The listing builds one solid part. Answer for the finished solid, in the listing's coordinates (mm). A direction names the side the tool comes from. Round coordinates to 2 decimals unless told otherwise and drop trailing zeros. Write each loop counter-clockwise with the first axis right and the second up, starting at its lowest first coordinate (ties: lowest second). Pieces come first, ordered by that corner, then holes. Notation, with made-up numbers: (56.25, 51) - (71.25, 51) arc R24 ccw to (71.25, 85) - close; hole circle Ø10 at (31, 24). An arc over 180 degrees is marked (long way). Answer in a Markdown table with one row per item.
from build123d import *

# Parameters (mm, degrees)
BOSS_EXTRUDE1_DEPTH                          = 75
SKETCH2_R                                    = 1.3
CUT_EXTRUDE1_DEPTH                           = 34
CBORE_FOR_M3_HEX_SOCKET_HEAD_CAP_SCR_2_COUNT = 2
CBORE_FOR_M3_HEX_SOCKET_HEAD_CAP_SCR_2_PITCH = 60
CBORE_FOR_M3_HEX_SOCKET_HEAD_CAP_SCR_3_COUNT = 2
CBORE_FOR_M3_HEX_SOCKET_HEAD_CAP_SCR_3_PITCH = 57.567351858
CBORE_FOR_M3_HEX_SOCKET_HEAD_CAP_SCR_4_COUNT = 2
CBORE_FOR_M3_HEX_SOCKET_HEAD_CAP_SCR_4_PITCH = 17.720045147
FILLET2_R                                    = 12.5
BOSS_EXTRUDE2_START                          = 10
BOSS_EXTRUDE2_DEPTH                          = 10
CHAMFER3_SIZE                                = 0.5
BOSS_EXTRUDE3_START                          = 1.5
BOSS_EXTRUDE3_DEPTH                          = 1.5


with BuildPart() as part:
    # Sketch1 → Boss-Extrude1 (new body)
    with BuildSketch(Plane.XY):
        Polygon((0, 0), (60, 0), (60, 8.5), (30, 8.5), (0, 8.5), align=None)
    extrude(amount=BOSS_EXTRUDE1_DEPTH)

    # Sketch2 → Cut-Extrude1 (cut)
    with BuildSketch(Plane(origin=(0, 8.5, 0), x_dir=(1, 0, 0), z_dir=(0, 1, 0))):
        with Locations(Location((45, -64.5, 0), (0, 0, 180))):
            Circle(SKETCH2_R)
        with Locations(Location((45, -10.5, 0), (0, 0, 180))):
            Circle(SKETCH2_R)
    extrude(amount=-CUT_EXTRUDE1_DEPTH, mode=Mode.SUBTRACT)

    # Sketch4 → CBORE for M3 Hex Socket Head Cap Screw1 (revolve, cut)
    with BuildSketch(Plane(origin=(25, 8.5, 67.5), x_dir=(0, 0, 1), z_dir=(1, 0, 0))):
        Polygon((0, 0), (0, 8.5), (1.825, 8.5), (1.8, 8.475), (1.8, 3.425), (1.825, 3.4), (3.25, 3.4), (3.25, 0.025), (3.275, 0), align=None)
    cbore_for_m3_hex_socket_head_cap_screw1 = revolve(axis=Axis((25, 14.85, 67.5), (0, -1, 0)), mode=Mode.SUBTRACT)

    # CBORE for M3 Hex Socket Head Cap Scr 2: CBORE for M3 Hex Socket Head Cap Screw1 ×2
    with Locations(*[(0, 0, -i * CBORE_FOR_M3_HEX_SOCKET_HEAD_CAP_SCR_2_PITCH) for i in range(1, CBORE_FOR_M3_HEX_SOCKET_HEAD_CAP_SCR_2_COUNT)]):
        add(cbore_for_m3_hex_socket_head_cap_screw1, mode=Mode.SUBTRACT)

    # CBORE for M3 Hex Socket Head Cap Scr 3: CBORE for M3 Hex Socket Head Cap Screw1 ×2
    with Locations(*[Vector(-0.2953062708492605, 0, -0.9554026409829016) * (i * CBORE_FOR_M3_HEX_SOCKET_HEAD_CAP_SCR_3_PITCH) for i in range(1, CBORE_FOR_M3_HEX_SOCKET_HEAD_CAP_SCR_3_COUNT)]):
        add(cbore_for_m3_hex_socket_head_cap_screw1, mode=Mode.SUBTRACT)

    # CBORE for M3 Hex Socket Head Cap Scr 4: CBORE for M3 Hex Socket Head Cap Screw1 ×2
    with Locations(*[Vector(-0.9593655015712707, 0, -0.28216632399155017) * (i * CBORE_FOR_M3_HEX_SOCKET_HEAD_CAP_SCR_4_PITCH) for i in range(1, CBORE_FOR_M3_HEX_SOCKET_HEAD_CAP_SCR_4_COUNT)]):
        add(cbore_for_m3_hex_socket_head_cap_screw1, mode=Mode.SUBTRACT)

    # Fillet2
    fillet2_edges = [part.edges().sort_by_distance(p)[0] for p in [
        (60, 4.25, 75),
        (0, 4.25, 75),
        (60, 4.25, 0),
        (0, 4.25, 0),
    ]]
    fillet(fillet2_edges, radius=FILLET2_R)

    # Sketch5 → Boss-Extrude2 (add)
    with BuildSketch(Plane(origin=(0, 8.5, 0), x_dir=(1, 0, 0), z_dir=(0, 1, 0)).offset(BOSS_EXTRUDE2_START)):
        with BuildLine():
            Line((47.5, 0), (42.5, 0))
            ThreePointArc((42.5, 0), (33.661165235, -3.661165235), (30, -12.5))
            Line((30, -12.5), (30, -62.5))
            ThreePointArc((30, -62.5), (33.661165235, -71.338834765), (42.5, -75))
            Line((42.5, -75), (47.5, -75))
            ThreePointArc((47.5, -75), (56.338834765, -71.338834765), (60, -62.5))
            Line((60, -62.5), (60, -12.5))
            ThreePointArc((60, -12.5), (56.338834765, -3.661165235), (47.5, 0))
        make_face()
        with BuildLine():
            Line((47.5, -2), (42.5, -2))
            ThreePointArc((42.5, -2), (35.075378798, -5.075378798), (32, -12.5))
            Line((32, -12.5), (32, -62.5))
            ThreePointArc((32, -62.5), (35.075378798, -69.924621202), (42.5, -73))
            Line((42.5, -73), (47.5, -73))
            ThreePointArc((47.5, -73), (54.924621202, -69.924621202), (58, -62.5))
            Line((58, -62.5), (58, -12.5))
            ThreePointArc((58, -12.5), (54.924621202, -5.075378798), (47.5, -2))
        make_face(mode=Mode.SUBTRACT)
    extrude(amount=-BOSS_EXTRUDE2_DEPTH)

    # Chamfer3
    chamfer3_edges = [part.edges().sort_by_distance(p)[0] for p in [
        (27.5, 8.5, 0),
        (27.5, 8.5, 75),
        (33.661165235, 18.5, 3.661165235),
        (30, 18.5, 37.5),
        (33.661165235, 18.5, 71.338834765),
        (45, 18.5, 75),
        (56.338834765, 18.5, 71.338834765),
        (60, 18.5, 37.5),
        (56.338834765, 18.5, 3.661165235),
        (45, 18.5, 0),
        (35.075378798, 18.5, 69.924621202),
        (45, 18.5, 73),
        (54.924621202, 18.5, 69.924621202),
        (58, 18.5, 37.5),
        (54.924621202, 18.5, 5.075378798),
        (45, 18.5, 2),
        (35.075378798, 18.5, 5.075378798),
        (32, 18.5, 37.5),
        (0, 0, 37.5),
        (0, 8.5, 37.5),
        (30, 0, 0),
        (60, 0, 37.5),
        (30, 0, 75),
        (56.338834765, 0, 71.338834765),
        (56.338834765, 0, 3.661165235),
        (3.661165235, 0, 71.338834765),
        (3.661165235, 0, 3.661165235),
        (3.661165235, 8.5, 71.338834765),
        (3.661165235, 8.5, 3.661165235),
    ]]
    chamfer(chamfer3_edges, length=CHAMFER3_SIZE)

    # Sketch6 → Boss-Extrude3 (add)
    with BuildSketch(Plane(origin=(0, 8.5, 0), x_dir=(1, 0, 0), z_dir=(0, 1, 0)).offset(BOSS_EXTRUDE3_START)):
        with BuildLine():
            Line((50.662375826, -16.5), (58, -16.5))
            Line((58, -16.5), (58, -12.5))
            ThreePointArc((58, -12.5), (54.924621202, -5.075378798), (47.5, -2))
            Line((47.5, -2), (42.5, -2))
            ThreePointArc((42.5, -2), (35.075378798, -5.075378798), (32, -12.5))
            Line((32, -12.5), (32, -16.5))
            Line((32, -16.5), (39.337624174, -16.5))
            ThreePointArc((39.337624174, -16.5), (41.732898882, -2.924476897), (53.25, -10.5))
            ThreePointArc((53.25, -10.5), (52.575523103, -13.767101118), (50.662375826, -16.5))
        make_face()
        with BuildLine():
            Line((58, -62.5), (58, -58.5))
            Line((58, -58.5), (50.662375826, -58.5))
            ThreePointArc((50.662375826, -58.5), (52.575523103, -61.232898882), (53.25, -64.5))
            ThreePointArc((53.25, -64.5), (41.732898882, -72.075523103), (39.337624174, -58.5))
            Line((39.337624174, -58.5), (32, -58.5))
            Line((32, -58.5), (32, -62.5))
            ThreePointArc((32, -62.5), (35.075378798, -69.924621202), (42.5, -73))
            Line((42.5, -73), (47.5, -73))
            ThreePointArc((47.5, -73), (54.924621202, -69.924621202), (58, -62.5))
        make_face()
    extrude(amount=-BOSS_EXTRUDE3_DEPTH)


solid = part.part
(1) For faces 1 (the cylindrical face through (33.565, 13.07, 71.241)), 2 (the cylindrical face through (46.3, 4.31, 64.56)), 3 (the flat face through (36, 9, 16.5)), determine the directions among +Z, -Z, +X, -X, +Y, -Y from which every point of the face is accessible in a straight line to the end or side of a thin tool.
Checked values:
| item | result |
|---|---|
| face 1 | +Z, -X, +Y |
| face 2 | +Y, -Y |
| face 3 | +Y |
(2) Section A-A (y = 3) is taken. Give the vertices of the cut face in (x, z).
Checked values:
| item | result |
|---|---|
| outline | (0, 12.5) arc R12.5 ccw to (12.5, 0) - (47.5, 0) arc R12.5 ccw to (60, 12.5) - (60, 62.5) arc R12.5 ccw to (47.5, 75) - (12.5, 75) arc R12.5 ccw to (0, 62.5) - close; hole circle Ø3.6 at (8, 12.5); hole circle Ø3.6 at (8, 62.5); hole circle Ø3.6 at (25, 7.5); hole circle Ø3.6 at (25, 67.5); hole circle Ø2.6 at (45, 10.5); hole circle Ø2.6 at (45, 64.5) |
(3) Flat-ended cylindrical pins translate along their axes: pin 1 (4 mm diameter, centred on x = 8, z = 62.5, fed in from +Y); pin 2 (5 mm diameter, centred on x = 35, z = 20.5, fed in from +Y); pin 3 (5 mm diameter, centred on y = 14, z = 36, fed in from -X). Find the tip coordinate at first contact, or state that the pin passes through.
Checked values:
| item | result |
|---|---|
| pin 1 | stops at y = 5.1 |
| pin 2 | stops at y = 8.5 |
| pin 3 | stops at x = 30 |
(4) For a pull along Z with two mould halves and no side action, classify faces 4 (the cylindrical face through (55.01, 14.06, 5.16)), 5 (the conical face through (34.014, 18.365, 3.825)), 6 (the flat face through (30, 0, 37)) as pulls with the +Z half, pulls with the -Z half, needs draft (parallel to the pull), parting line crosses it, or undercut.
Checked values:
| item | result |
|---|---|
| face 4 | undercut |
| face 5 | pulls with the -Z half |
| face 6 | needs draft |
(5) Section C-C (z = 41) is taken. Give the vertices of the cut face in (x, y), and give its area (3 significant figures).
Checked values:
| item | result |
|---|---|
| outline | (0, 0.5) - (0.5, 0) - (59.5, 0) - (60, 0.5) - (60, 18) - (59.5, 18.5) - (58.5, 18.5) - (58, 18) - (58, 8.5) - (32, 8.5) - (32, 18) - (31.5, 18.5) - (30.5, 18.5) - (30, 18) - (30, 8.5) - (0.5, 8.5) - (0, 8) - close |
| area | 549 mm2 |
(6) Section D-D (y = 12.5) is taken. Give the vertices of the cut face in (x, z).
Checked values:
| item | result |
|---|---|
| outline | (30, 12.5) arc R12.5 ccw to (42.5, 0) - (47.5, 0) arc R12.5 ccw to (60, 12.5) - (60, 62.5) arc R12.5 ccw to (47.5, 75) - (42.5, 75) arc R12.5 ccw to (30, 62.5) - close; hole (32, 12.5) arc R10.5 ccw to (42.5, 2) - (47.5, 2) arc R10.5 ccw to (58, 12.5) - (58, 62.5) arc R10.5 ccw to (47.5, 73) - (42.5, 73) arc R10.5 ccw to (32, 62.5) - close |
(7) Find the intervals of material crossed by line 1 (Z direction, x = 25, y = 3.5); line 2 (Z direction, x = 45, y = 6); line 3 (X direction, y = 1.55, z = 62.5), in increasing order.
Checked values:
| item | result |
|---|---|
| line 1 | z = 0 to 5.7, 9.3 to 65.7, 69.3 to 75 |
| line 2 | z = 0 to 9.2, 11.8 to 63.2, 65.8 to 75 |
| line 3 | x = 0 to 6.2, 9.8 to 60 |
(8) Section B-B (x = 45) is taken. Give the vertices of the cut face in (y, z).
Checked values:
| item | result |
|---|---|
| outline | (0, 0.5) - (0.5, 0) - (18, 0) - (18.5, 0.5) - (18.5, 1.5) - (18, 2) - (10, 2) - (10, 2.25) - (8.5, 2.25) - (8.5, 9.2) - (0, 9.2) - close; (0, 11.8) - (8.5, 11.8) - (8.5, 63.2) - (0, 63.2) - close; (0, 65.8) - (8.5, 65.8) - (8.5, 72.75) - (10, 72.75) - (10, 73) - (18, 73) - (18.5, 73.5) - (18.5, 74.5) - (18, 75) - (0.5, 75) - (0, 74.5) - close |
